Answer from the drawing. Dimensions are ordinates in mm from the lowest x, y and z of the part. A direction names the side the tool comes from. Round coordinates to 2 decimals unless told otherwise and drop trailing zeros. Loops run counter-clockwise (first coordinate to the right, second up) from the corner with the lowest first, then second, coordinate; pieces in that order, holes last. Notation, with made-up numbers: M 47.5,29.5 L 54.5,29.5 A11 cw 54.5,37.5 Z; hole C 74.25,-16.5 d9. An arc over 180 degrees is marked long. Write each question's results on one line, items separated by ' | '.
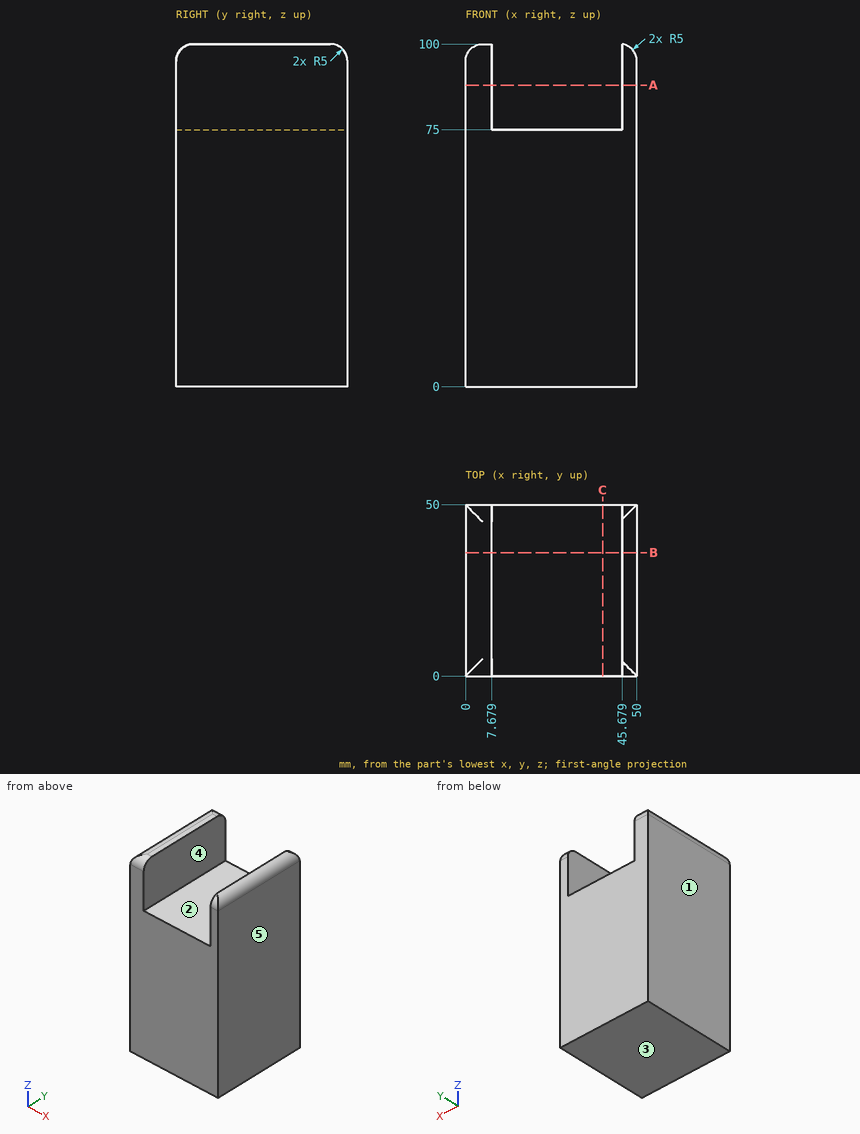
1. Determine the mould class of the marked faces 1, 2 and 3 for opening direction X: released by +X, released by -X, zero draft, split by the parting line, or undercut.
Completed:
face 1: released by -X | face 2: undercut | face 3: zero draft
2. Find section A-A, the plane z = 88. Give the vertices of the cut face in (x, y).
Completed:
outline: M 0,0 L 7.68,0 L 7.68,50 L 0,50 Z; M 45.68,0 L 50,0 L 50,50 L 45.68,50 Z
3. Which of the six approach directions +Z, -Z, +X, -X, +Y, -Y give full straight-line access (tool end or side, diameter ignored) to the marked faces 4 and 5?
Completed:
face 4: +Z, +Y, -Y | face 5: +Z, -Z, +X, +Y, -Y
4. Find section C-C, the plane x = 40. Give the vertices of the cut face in (y, z).
Completed:
outline: M 0,0 L 50,0 L 50,75 L 0,75 Z
5. Given P1, Ø1.5, axis at y = 11.5, z = 81, coming from the -X side; P2, Ø12, axis at x = 18, y = 18.5, coming from the +Z side, each flat-ended and moving along its own axis, determine where each tip first touches the part or whether it passes through.
Completed:
P1: stops at x = 0 | P2: stops at z = 75
6. Find the intervals of material crossed by L1, parallel to X at y = 4, z = 85; L2, parallel to Z at x = 34.5, y = 30; L3, parallel to Z at x = 47, y = 23, in increasing order.
Completed:
L1: x = 0 to 7.68, 45.68 to 50 | L2: z = 0 to 75 | L3: z = 0 to 99.58
7. Find section B-B, the plane y = 36. Give the vertices of the cut face in (x, z), then the cut area to 3 significant figures.
Completed:
outline: M 0,0 L 50,0 L 50,95 A5 ccw 45.68,99.95 L 45.68,75 L 7.68,75 L 7.68,100 L 5,100 A5 ccw 0,95 Z | area: 4,040 mm2
